The model under review builds one solid part; all positions refer to its coordinate system, in mm. Face numbers are marked on the shaded views. A direction names the side the tool comes from. Round coordinates to 2 decimals unless told otherwise and drop trailing zeros. Loops run counter-clockwise (first coordinate to the right, second up) from the corner with the lowest first, then second, coordinate; pieces in that order, holes last. Notation, with made-up numbers: M 86.25,14.25 L 109.25,14.25 A29 cw 109.25,37.25 Z; hole C 18,48.5 d7. An arc over 180 degrees is marked long. Return JSON: item names as keys, results as strings. Group by question number.
Q1. Consider section C-C (z = -11.75). State the section outline as (x, y) points, and give its area (4 significant figures).
Q2. Draft analysis for pull direction X (two halves, no side actions). For the marked faces 5, 6 and 7, state which applies: pulls with the +X half, pulls with the -X half, needs draft (parallel to the pull), parting line crosses it, or undercut.
Q3. Consider section B-B (x = 9.5). State the section outline as (y, z) points, and give its area (4 significant figures).
Q4. For the marked faces 1, 2, 3 and 4, list the 3-axis set-ups (+Z, -Z, +X, -X, +Y, -Y) from which the entire face can be reached by the end or side of a thin tool; tool diameter is ignored.
Q5. Clearance check with flat-ended pins moving along their axes: pin 1 Ø1 at (y, z) = (14, -13) entering from +X; pin 2 Ø4 at (x, y) = (8, 18) entering from +Z; pin 3 Ø2 at (y, z) = (22.5, -2) entering from -X. State where each tip first meets the part, or that it passes through.
Q6. To check wall thickness, follow line 1 along Z through (x, y) = (6.5, 26.4); line 2 along X through (y, z) = (25.85, -7.5); line 3 along X through (y, z) = (17.25, -10.25). State the ranges of each line that lie inside material, in increasing order.
Q7. Consider section A-A (z = -7.5). State the section outline as (x, y) points, and give its area (4 significant figures).
Q8. Consider section D-D (y = 14.5). State the section outline as (x, z) points.
from build123d import *

# Parameters (mm, degrees)
SKETCH1_W           = 13
SKETCH1_H           = 15
BOSS_EXTRUDE1_DEPTH = 10
SKETCH2_W           = 8.5
SKETCH2_H           = 10.5
BOSS_EXTRUDE2_DEPTH = 17
SKETCH3_R           = 2.25
CUT_EXTRUDE1_DEPTH  = 2


with BuildPart() as part:
    # Sketch1 → Boss-Extrude1 (new body)
    with BuildSketch(Plane(origin=(0, 0, 0), x_dir=(1, 0, 0), z_dir=(0, 1, 0))):
        with Locations((6.5, 7.5)):
            Rectangle(SKETCH1_W, SKETCH1_H)
    extrude(amount=BOSS_EXTRUDE1_DEPTH)

    # Sketch2 → Boss-Extrude2 (add)
    with BuildSketch(Plane(origin=(0, 10, 0), x_dir=(1, 0, 0), z_dir=(0, 1, 0))):
        with Locations((6.5, 7.5)):
            Rectangle(SKETCH2_W, SKETCH2_H)
    extrude(amount=BOSS_EXTRUDE2_DEPTH)

    # Sketch3 → Cut-Extrude1 (cut)
    with BuildSketch(Plane(origin=(0, 27, 0), x_dir=(1, 0, 0), z_dir=(0, 1, 0))):
        with Locations((6.5, 7.5)):
            Circle(SKETCH3_R)
    extrude(amount=-CUT_EXTRUDE1_DEPTH, mode=Mode.SUBTRACT)


solid = part.part
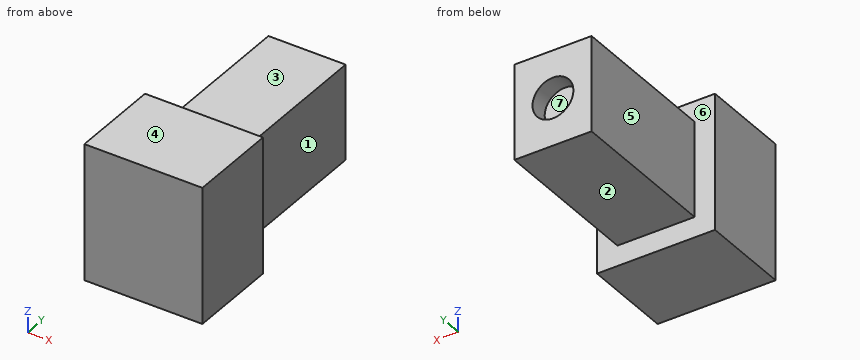
Values:
{
 "1": {"outline": "M 0,0 L 13,0 L 13,10 L 10.75,10 L 10.75,27 L 2.25,27 L 2.25,10 L 0,10 Z", "area": "274.5 mm2"},
 "2": {"face 5": "pulls with the -X half", "face 6": "needs draft", "face 7": "undercut"},
 "3": {"outline": "M 0,-15 L 10,-15 L 10,-12.75 L 27,-12.75 L 27,-2.25 L 10,-2.25 L 10,0 L 0,0 Z", "area": "328.5 mm2"},
 "4": {"face 1": "+Z, -Z, +X, +Y", "face 2": "-Z, +X, -X, +Y", "face 3": "+Z, +X, -X, +Y", "face 4": "+Z, +X, -X, +Y, -Y"},
 "5": {"pin 1": "stops at x = 10.75", "pin 2": "stops at z = -2.25", "pin 3": "stops at x = 2.25"},
 "6": {"line 1": "z = -12.75 to -9.75, -5.25 to -2.25", "line 2": "x = 2.25 to 4.25, 8.75 to 10.75", "line 3": "x = 2.25 to 10.75"},
 "7": {"outline": "M 0,0 L 13,0 L 13,10 L 10.75,10 L 10.75,27 L 8.75,27 L 8.75,25 L 4.25,25 L 4.25,27 L 2.25,27 L 2.25,10 L 0,10 Z", "area": "265.5 mm2"},
 "8": {"outline": "M 2.25,-12.75 L 10.75,-12.75 L 10.75,-2.25 L 2.25,-2.25 Z"}
}
